from build123d import *

# Parameters (mm, degrees)
ESQUISSE1_W             = 20
ESQUISSE1_H             = 40
BOSS_EXTRU_1_DEPTH      = 3
ENL_V_MAT_EXTRU_1_REACH = 5
ESQUISSE2_R             = 2
ESQUISSE2_W             = 8.5
ESQUISSE2_H             = 5
ESQUISSE2_W_2           = 5
ESQUISSE2_H_2           = 7
ENL_V_MAT_EXTRU_2_REACH = 5
ESQUISSE3_W             = 14
ESQUISSE3_H             = 5
ESQUISSE3_H_2           = 6


with BuildPart() as part:
    # Esquisse1 → Boss.-Extru.1 (new body)
    with BuildSketch(Plane.XY):
        with Locations((10, 20)):
            Rectangle(ESQUISSE1_W, ESQUISSE1_H)
    extrude(amount=BOSS_EXTRU_1_DEPTH)

    # Esquisse2 → Enlèv. mat.-Extru.1 (cut, up to next)
    with BuildSketch(Plane.XY.offset(3), mode=Mode.PRIVATE) as enl_v_mat_extru_1_sk1:
        with Locations((10, 20)):
            Circle(ESQUISSE2_R)
    enl_v_mat_extru_1_tool1 = extrude(enl_v_mat_extru_1_sk1.sketch, amount=-ENL_V_MAT_EXTRU_1_REACH, mode=Mode.PRIVATE) & part.part
    add(enl_v_mat_extru_1_tool1.solids().sort_by_distance((10, 20, 3))[0], mode=Mode.SUBTRACT)
    # Esquisse2 → Enlèv. mat.-Extru.1 (cut, up to next)
    with BuildSketch(Plane.XY.offset(3), mode=Mode.PRIVATE) as enl_v_mat_extru_1_sk2:
        with Locations((10, 29)):
            Rectangle(ESQUISSE2_W, ESQUISSE2_H)
    enl_v_mat_extru_1_tool2 = extrude(enl_v_mat_extru_1_sk2.sketch, amount=-ENL_V_MAT_EXTRU_1_REACH, mode=Mode.PRIVATE) & part.part
    add(enl_v_mat_extru_1_tool2.solids().sort_by_distance((10, 29, 3))[0], mode=Mode.SUBTRACT)
    # Esquisse2 → Enlèv. mat.-Extru.1 (cut, up to next)
    with BuildSketch(Plane.XY.offset(3), mode=Mode.PRIVATE) as enl_v_mat_extru_1_sk3:
        with Locations((10, 11)):
            Rectangle(ESQUISSE2_W_2, ESQUISSE2_H_2)
    enl_v_mat_extru_1_tool3 = extrude(enl_v_mat_extru_1_sk3.sketch, amount=-ENL_V_MAT_EXTRU_1_REACH, mode=Mode.PRIVATE) & part.part
    add(enl_v_mat_extru_1_tool3.solids().sort_by_distance((10, 11, 3))[0], mode=Mode.SUBTRACT)

    # Esquisse3 → Enlèv. mat.-Extru.2 (cut, up to next)
    with BuildSketch(Plane.XY.offset(3), mode=Mode.PRIVATE) as enl_v_mat_extru_2_sk1:
        Polygon((0, 40), (0, 0), (3, 0), (3, 5), (3, 34), (3, 40), align=None)
    enl_v_mat_extru_2_tool1 = extrude(enl_v_mat_extru_2_sk1.sketch, amount=-ENL_V_MAT_EXTRU_2_REACH, mode=Mode.PRIVATE) & part.part
    add(enl_v_mat_extru_2_tool1.solids().sort_by_distance((1.5, 20, 3))[0], mode=Mode.SUBTRACT)
    # Esquisse3 → Enlèv. mat.-Extru.2 (cut, up to next)
    with BuildSketch(Plane.XY.offset(3), mode=Mode.PRIVATE) as enl_v_mat_extru_2_sk2:
        Polygon((17, 5), (17, 0), (20, 0), (20, 40), (17, 40), (17, 34), align=None)
    enl_v_mat_extru_2_tool2 = extrude(enl_v_mat_extru_2_sk2.sketch, amount=-ENL_V_MAT_EXTRU_2_REACH, mode=Mode.PRIVATE) & part.part
    add(enl_v_mat_extru_2_tool2.solids().sort_by_distance((18.5, 20, 3))[0], mode=Mode.SUBTRACT)
    # Esquisse3 → Enlèv. mat.-Extru.2 (cut, up to next)
    with BuildSketch(Plane.XY.offset(3), mode=Mode.PRIVATE) as enl_v_mat_extru_2_sk3:
        with Locations((10, 2.5)):
            Rectangle(ESQUISSE3_W, ESQUISSE3_H)
    enl_v_mat_extru_2_tool3 = extrude(enl_v_mat_extru_2_sk3.sketch, amount=-ENL_V_MAT_EXTRU_2_REACH, mode=Mode.PRIVATE) & part.part
    add(enl_v_mat_extru_2_tool3.solids().sort_by_distance((10, 2.5, 3))[0], mode=Mode.SUBTRACT)
    # Esquisse3 → Enlèv. mat.-Extru.2 (cut, up to next)
    with BuildSketch(Plane.XY.offset(3), mode=Mode.PRIVATE) as enl_v_mat_extru_2_sk4:
        with Locations((10, 37)):
            Rectangle(ESQUISSE3_W, ESQUISSE3_H_2)
    enl_v_mat_extru_2_tool4 = extrude(enl_v_mat_extru_2_sk4.sketch, amount=-ENL_V_MAT_EXTRU_2_REACH, mode=Mode.PRIVATE) & part.part
    add(enl_v_mat_extru_2_tool4.solids().sort_by_distance((10, 37, 3))[0], mode=Mode.SUBTRACT)


solid = part.part
Input: part model. Units: mm. Frame: model coordinates. A direction names the side the tool comes from. Give positions to 0.01 mm unless a question says otherwise; leave off trailing zeros. Order: outer loops, then holes, each group sorted by start corner. A loop starts at its lowest first (then second) coordinate and runs counter-clockwise, first axis right, second up. Notation, with made-up numbers: (40, 69.5) - (65, 69.5) arc R20 ccw to (65, 106.5) - close; hole circle Ø1 at (0, -1). An arc over 180 degrees is marked (long way). Answer as a JSON object with one key per item and string values. Group by question number.
Q1. Line query: probe 1 along Y at (x, z) = (10, 1.85); probe 2 along X at (y, z) = (28, 1.05); probe 3 along X at (y, z) = (11, 1.8). Output: solid intervals per line, ascending.
Q2. Cut plane B-B, the plane x = 10. Output: boundary loops of the cut face in (y, z).
Q3. Cut plane C-C, the plane z = 2.1. Output: boundary loops of the cut face in (x, y).
Q4. Cut plane A-A, the plane y = 20. Output: boundary loops of the cut face in (x, z), then the cut area to 3 significant figures.
Q5. Set-up query: faces 4 (the face through (7, 20, 0)), 5 (the face through (5.75, 29, 2)). Return all of +Z, -Z, +X, -X, +Y, -Y with unobstructed straight access to the full face (end or side cutting, diameter ignored); none if empty.
Q6. Mould query, pull axis Y, two halves, no side actions, for faces 1 (the face through (7, 20, 3)), 2 (the face through (12.5, 11, 2)), 3 (the face through (10, 34, 2)). Classes: pulls with the +Y half, pulls with the -Y half, needs draft (parallel to the pull), parting line crosses it, or undercut.
Q7. First-contact query: pin 1 Ø5 at (x, y) = (10, 20) entering from -Z; pin 2 Ø2 at (x, y) = (10.5, 10) entering from -Z. Flat tips, straight axial feed; report the tip coordinate or a pass-through.
Q8. Cut plane D-D, the plane y = 29.25. Output: boundary loops of the cut face in (x, z).
Results:
{
 "1": {"probe 1": "5 to 7.5, 14.5 to 18, 22 to 26.5, 31.5 to 34", "probe 2": "3 to 5.75, 14.25 to 17", "probe 3": "3 to 7.5, 12.5 to 17"},
 "2": {"outline": "(5, 0) - (7.5, 0) - (7.5, 3) - (5, 3) - close; (14.5, 0) - (18, 0) - (18, 3) - (14.5, 3) - close; (22, 0) - (26.5, 0) - (26.5, 3) - (22, 3) - close; (31.5, 0) - (34, 0) - (34, 3) - (31.5, 3) - close"},
 "3": {"outline": "(3, 5) - (17, 5) - (17, 34) - (3, 34) - close; hole (5.75, 26.5) - (14.25, 26.5) - (14.25, 31.5) - (5.75, 31.5) - close; hole (7.5, 7.5) - (12.5, 7.5) - (12.5, 14.5) - (7.5, 14.5) - close; hole circle Ø4 at (10, 20)"},
 "4": {"outline": "(3, 0) - (8, 0) - (8, 3) - (3, 3) - close; (12, 0) - (17, 0) - (17, 3) - (12, 3) - close", "area": "30.0 mm^2"},
 "5": {"face 4": "-Z, +X, -X, +Y, -Y", "face 5": "+Z, -Z"},
 "6": {"face 1": "needs draft", "face 2": "undercut", "face 3": "pulls with the +Y half"},
 "7": {"pin 1": "z = 0", "pin 2": "through"},
 "8": {"outline": "(3, 0) - (5.75, 0) - (5.75, 3) - (3, 3) - close; (14.25, 0) - (17, 0) - (17, 3) - (14.25, 3) - close"}
}
